Could you check a few things on this model? Use its own coordinates, in mm. A direction names the side the tool comes from. Coordinates: 2 decimals unless noted, no trailing zeros. Loops run counter-clockwise (first coordinate to the right, second up) from the corner with the lowest first, then second, coordinate; pieces in that order, holes last. Notation, with made-up numbers: (84, 63) -> (110, 63) arc R10 ccw to (110, 82) -> close; hole circle Ø10 at (54, 89). An arc over 180 degrees is marked (long way). One line per question, with ' | ' between items.
Autodesk Fusion 360 part; units mm, degrees
sketch "Sketch1" plane through (0, 0, 0) normal (0, 0, 1) x (1, 0, 0)
  line L0 (0, -33) -> (94, -33)
  arc A0 (94, -33) -> (94, 33) centre (94, 0) ccw
  line L1 (94, 33) -> (0, 33)
  arc A1 (0, 33) -> (0, -33) centre (0, 0) ccw
  line L2 (0, 0) -> (94, 0) construction
  point P0 (-33, 0)
  point P1 (127, 0)
  dimension "d1" = 94
  dimension "d2" = 66
  dimension "d3" = 33
  dimension "d4" = 160
extrude "Extrude1" add sketch "Sketch1" along normal blind 40
move_face "OffsetFaces1" offset 5 1 faces at (62.6667, -11, 40)
sketch "Sketch2" plane through (0, 0, 45) normal (0, 0, 1) x (-1, 0, 0)
  arc A0 (0, -33) -> (0, 33) centre (0, 0) ccw
  line L0 (0, 33) -> (-94, 33)
  arc A1 (-94, 33) -> (-94, -33) centre (-94, 0) ccw
  line L1 (-94, -33) -> (0, -33)
  line L2 (0, 29) -> (-94, 29)
  arc A2 (-94, 29) -> (-94, -29) centre (-94, 0) ccw
  line L3 (-94, -29) -> (0, -29)
  arc A3 (0, -29) -> (0, 29) centre (0, 0) ccw
  dimension "d8" = -4
extrude "Extrude2" cut sketch "Sketch2" against normal blind 40 contours L2 A2 L3 A3
sketch "Sketch3" plane through (0, 0, 5) normal (0, 0, 1) x (-1, 0, 0)
  arc A0 (0, -29) -> (0, 29) centre (0, 0) ccw
  line L0 (0, 29) -> (-94, 29)
  arc A1 (-94, 29) -> (-94, -29) centre (-94, 0) ccw
  line L1 (-94, -29) -> (0, -29)
  line L2 (0, 27) -> (-94, 27)
  arc A2 (-94, 27) -> (-94, -27) centre (-94, 0) ccw
  line L3 (-94, -27) -> (0, -27)
  arc A3 (0, -27) -> (0, 27) centre (0, 0) ccw
  dimension "d11" = -2
sketch "Sketch4" plane through (0, 0, 5) normal (0, 0, 1) x (-1, 0, 0)
  arc A0 (0, -29) -> (0, 29) centre (0, 0) ccw
  line L0 (0, 29) -> (-94, 29)
  arc A1 (-94, 29) -> (-94, -29) centre (-94, 0) ccw
  line L1 (-94, -29) -> (0, -29)
extrude "Extrude3" add sketch "Sketch3" along normal blind 2
move_face "MoveFace1" by (0, 0, 30) 1 faces at (31.3333, 28.3333, 7)
move_face "MoveFace2" by (0, 0, 7.8672) 1 faces at (31.3333, 28.3333, 37)
move_face "MoveFace3" by (0, 0, 0.08) 1 faces at (31.3333, 28.3333, 44.8672)
move_face "MoveFace4" by (0, 0, 0.05) 1 faces at (31.3333, 28.3333, 44.9472)
move_face "MoveFace5" by (0, -5, -2.8) 1 faces at (31.3333, 28.3333, 44.9972)
sketch "Sketch5" plane through (0, 0, 0) normal (0, 0, 1) x (1, 0, 0)
sketch "Sketch6" plane through (0, 0, 0) normal (0, 0, 1) x (1, 0, 0)
  line L0 (-20, 10) -> (35, 10)
  line L1 (35, 10) -> (35, -20)
  line L2 (35, -20) -> (-20, -20)
  line L3 (-20, -20) -> (-20, 10)
sketch "Sketch8" plane through (0, 0, 0) normal (0, 0, -1) x (1, 0, 0)
  arc A0 (0, 33) -> (0, -33) centre (0, 0) ccw
  line L0 (0, -33) -> (94, -33)
  arc A1 (94, -33) -> (94, 33) centre (94, 0) ccw
  line L1 (94, 33) -> (0, 33)
sketch "Sketch9" plane through (0, -33, 0) normal (0, -1, 0) x (1, 0, 0)
  line L0 (0, 0) -> (94, 0)
  line L1 (94, 0) -> (94, 45)
  line L2 (94, 45) -> (0, 45)
  line L3 (0, 45) -> (0, 0)
  line L4 (75, 25) -> (81.5, 25)
  line L5 (81.5, 25) -> (81.5, 18.5)
  line L6 (81.5, 18.5) -> (75, 18.5)
  line L7 (75, 18.5) -> (75, 25)
  dimension "d22" = 6.5
  dimension "d23" = 6.5
extrude "Extrude7" cut sketch "Sketch9" against normal blind 15 contours L4 L5 L6 L7
1) We'd pull the mould along Y, two halves only. Please class faces 4 (the face through (126.99, 0.73, 22.18)), 5 (the face through (48, 33, 22)), 6 (the face through (48, 29, 44)): pulls with the +Y half, pulls with the -Y half, needs draft (parallel to the pull), parting line crosses it, or undercut.
Data:
face 4: parting line crosses it | face 5: pulls with the +Y half | face 6: undercut
2) I need wall thicknesses on line 1 along Y through (x, z) = (80.5, 38.5); line 2 along Z through (x, y) = (38.5, -6.5); line 3 along X through (y, z) = (19, 41.5). Which ranges of each line are inside material? Lowest first, please. Write a range as from..to.
Data:
line 1: -33..-27, 27..33 | line 2: 0..5 | line 3: -26.98..-19.18, 113.18..120.98
3) If we section it at A-A on y = 0: Please give me the cut outline in (x, z).
Data:
outline: (-33, 0) -> (127, 0) -> (127, 45) -> (123, 45) -> (123, 42.2) -> (121, 42.2) -> (121, 5) -> (-27, 5) -> (-27, 42.2) -> (-29, 42.2) -> (-29, 45) -> (-33, 45) -> close
4) I'm going to push flat-ended pins straight in: pin 1 Ø6 at (x, y) = (3.5, -25) entering from +Z; pin 2 Ø2 at (y, z) = (10.5, 32.5) entering from +X; pin 3 Ø3 at (x, z) = (-14, 10) entering from +Y. Where does each tip first touch, or does it pass through?
Data:
pin 1: z = 42.2 | pin 2: x = 125.6 | pin 3: y = 30.54
5) If we section it at B-B on x = 90: Please give me the cut outline in (y, z).
Data:
outline: (-33, 0) -> (33, 0) -> (33, 45) -> (29, 45) -> (29, 42.2) -> (27, 42.2) -> (27, 5) -> (-27, 5) -> (-27, 42.2) -> (-29, 42.2) -> (-29, 45) -> (-33, 45) -> close
6) On a 3-axis mill with a long thin cutter (end or side, diameter ignored), from which of +Z, -Z, +X, -X, +Y, -Y can I reach the whole of each face in a straight line? I mean faces 1 (the face through (-26.993, -0.594, 23.338)), 2 (the face through (75, -30, 22)), 3 (the face through (46, 0, 0)). Say none if no direction works.
Data:
face 1: +Z | face 2: -Y | face 3: -Z, +X, -X, +Y, -Y
